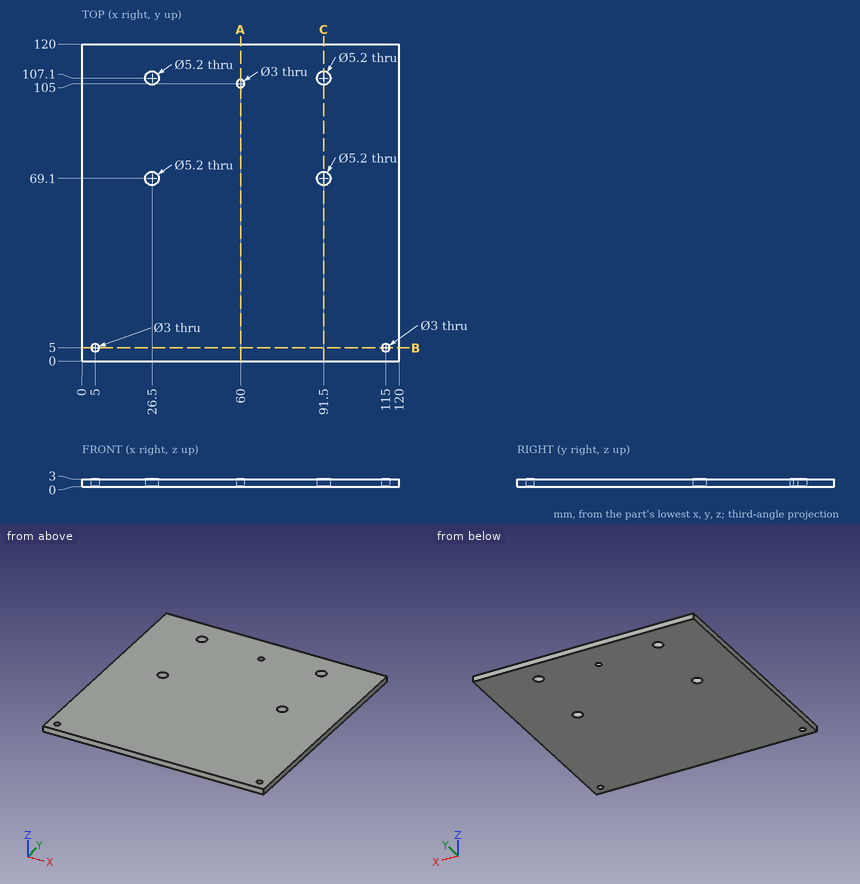
Design review of the part shown in the three views and the two pictorial views. Dimensions are in mm from the part's minimum x, y and z. Give positions to 0.01 mm unless a question says otherwise; leave off trailing zeros. Loops run counter-clockwise (first coordinate to the right, second up) from the corner with the lowest first, then second, coordinate; pieces in that order, holes last. Notation, with made-up numbers: M 69,-9 L 113,-9 A16 cw 113,16 Z; hole C -16.75,-29 d8. An arc over 180 degrees is marked long. Answer as a JSON object with one key per item and string values. Group by question number.
Q1. Insertion check: P1, Ø3, axis at x = 26.5, y = 107.1, coming from the -Z side. The pin has a flat end and moves straight along its axis. Give the tip position at first contact, or say it passes through.
Q2. Add section B-B on y = 5. Give the boundary of the cut face in (x, z).
Q3. For probe 1 along X at (y, z) = (69.1, 0.7); probe 2 along Y at (x, z) = (5, 2.35), list the stretches that pass through material, from the lowest coordinate up. Write a range as [from, to].
Q4. Add section C-C on x = 91.5. Give the boundary of the cut face in (y, z), and give its area (3 significant figures).
Q5. Add section A-A on x = 60. Give the boundary of the cut face in (y, z).
Checked values:
{
 "1": {"P1": "through"},
 "2": {"outline": "M 0,0 L 3.5,0 L 3.5,3 L 0,3 Z; M 6.5,0 L 113.5,0 L 113.5,3 L 6.5,3 Z; M 116.5,0 L 120,0 L 120,3 L 116.5,3 Z"},
 "3": {"probe 1": "[0, 23.9], [29.1, 88.9], [94.1, 120]", "probe 2": "[0, 3.5], [6.5, 120]"},
 "4": {"outline": "M 0,0 L 66.5,0 L 66.5,3 L 0,3 Z; M 71.7,0 L 104.5,0 L 104.5,3 L 71.7,3 Z; M 109.7,0 L 120,0 L 120,3 L 109.7,3 Z", "area": "329 mm²"},
 "5": {"outline": "M 0,0 L 103.5,0 L 103.5,3 L 0,3 Z; M 106.5,0 L 120,0 L 120,3 L 106.5,3 Z"}
}
